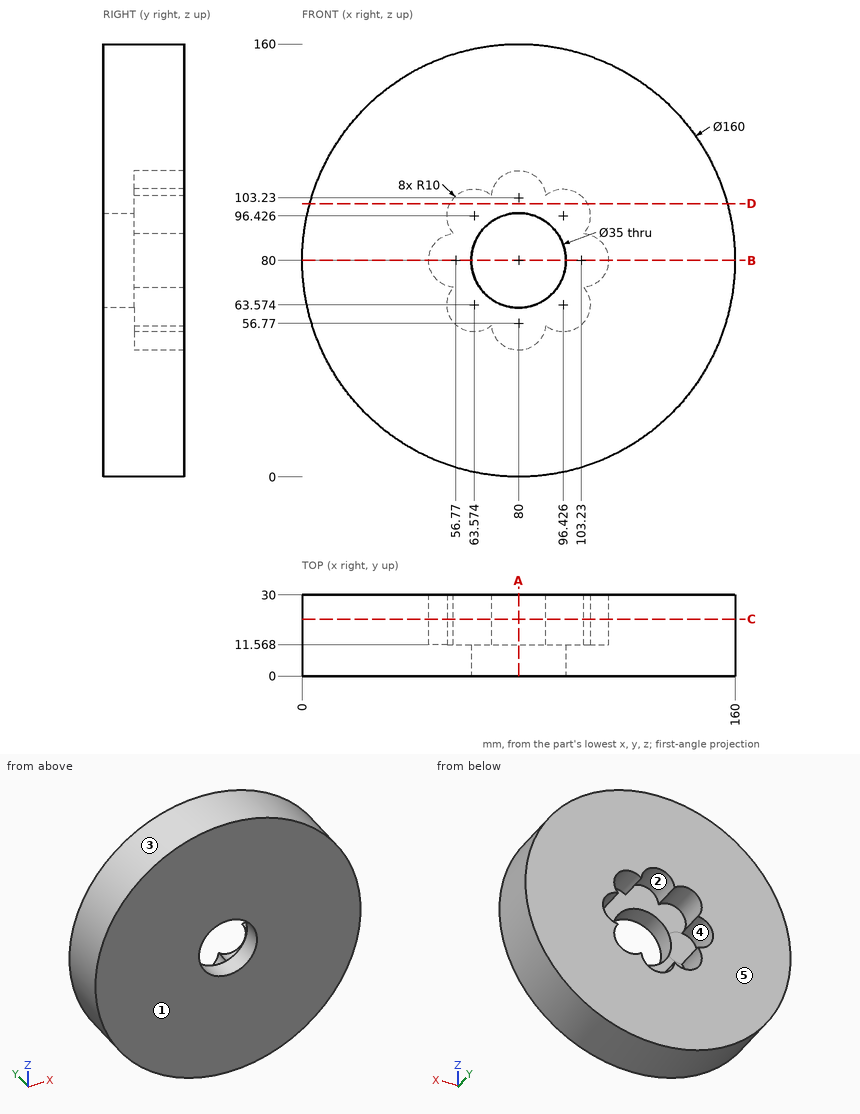
The drawing under review shows one solid part. Ordinate dimensions are in mm from its lowest x, y, z. A direction names the side the tool comes from. Round coordinates to 2 decimals unless told otherwise and drop trailing zeros. Loops run counter-clockwise (first coordinate to the right, second up) from the corner with the lowest first, then second, coordinate; pieces in that order, holes last.
Item 1: Take a section at C-C (y = 21). Write out the cut boundary in (x, z).
Determined:
outline: circle Ø160 at (80, 80); hole (55.94, 70.03) arc R10 ccw to (70.03, 55.94) arc R10 ccw to (89.97, 55.94) arc R10 ccw to (104.06, 70.03) arc R10 ccw to (104.06, 89.97) arc R10 ccw to (89.97, 104.06) arc R10 ccw to (70.03, 104.06) arc R10 ccw to (55.94, 89.97) arc R10 ccw to start
Item 2: For the marked faces 4 and 5, list the 3-axis set-ups (+Z, -Z, +X, -X, +Y, -Y) from which the entire face can be reached by the end or side of a thin tool; tool diameter is ignored.
Determined:
face 4: +Y
face 5: +Z, -Z, +X, -X, +Y
Item 3: Mouldability with a two-part tool opening along X and no side actions: class the marked faces 1, 2 and 3 as released by +X, released by -X, zero draft, split by the parting line, or undercut.
Determined:
face 1: zero draft
face 2: undercut
face 3: split by the parting line
Item 4: Take a section at D-D (z = 101). Write out the cut boundary in (x, y).
Determined:
outline: (2.81, 0) - (157.19, 0) - (157.19, 30) - (105.32, 30) - (105.32, 11.57) - (54.68, 11.57) - (54.68, 30) - (2.81, 30) - close
Item 5: For line 1 (X direction, y = 8, z = 80); line 2 (X direction, y = 4.75, z = 70); line 3 (Z direction, x = 62, y = 20.5), list the stretches that pass through material, from the lowest coordinate up.
Determined:
line 1: x = 0 to 62.5, 97.5 to 160
line 2: x = 0.63 to 65.64, 94.36 to 159.37
line 3: z = 2.05 to 53.7, 106.3 to 157.95
Item 6: Take a section at B-B (z = 80). Write out the cut boundary in (x, y), then the cut area to 3 significant figures.
Determined:
outline: (0, 0) - (62.5, 0) - (62.5, 11.57) - (46.77, 11.57) - (46.77, 30) - (0, 30) - close; (97.5, 0) - (160, 0) - (160, 30) - (113.23, 30) - (113.23, 11.57) - (97.5, 11.57) - close
area: 3,170 mm2
Item 7: Clearance check with flat-ended pins moving along their axes: pin 1 Ø8 at (y, z) = (21.5, 69) entering from +X; pin 2 Ø4 at (x, y) = (103, 10.5) entering from -Z; pin 3 Ø1.5 at (x, y) = (55, 17) entering from +Z. State where each tip first meets the part, or that it passes through.
Determined:
pin 1: stops at x = 159.69
pin 2: stops at z = 2.81
pin 3: stops at z = 156.24
Item 8: Take a section at A-A (x = 80). Write out the cut boundary in (y, z), then the cut area to 3 significant figures.
Determined:
outline: (0, 0) - (30, 0) - (30, 46.77) - (11.57, 46.77) - (11.57, 62.5) - (0, 62.5) - close; (0, 97.5) - (11.57, 97.5) - (11.57, 113.23) - (30, 113.23) - (30, 160) - (0, 160) - close
area: 3,170 mm2
